from build123d import *

# Parameters (mm, degrees)
SKETCH_R  = 3
PAD_DEPTH = 5


with BuildPart() as part:
    # Sketch → Pad (new body)
    with BuildSketch(Plane.XY):
        with BuildLine():
            Line((3, 43), (3, 13))
            Line((3, 13), (-3, 13))
            Line((-3, 13), (-3, 43))
            Line((-3, 43), (-8, 43))
            ThreePointArc((-43, 8), (-18.530637, 18.530637), (-8, 43))
            Line((-43, 3), (-43, 8))
            Line((-13, 3), (-43, 3))
            Line((-13, -3), (-13, 3))
            Line((-43, -3), (-13, -3))
            Line((-43, -3), (-43, -8))
            ThreePointArc((-8, -43), (-18.530637, -18.530637), (-43, -8))
            Line((-3, -43), (-8, -43))
            Line((-3, -43), (-3, -13))
            Line((-3, -13), (3, -13))
            Line((3, -13), (3, -43))
            Line((3, -43), (8, -43))
            ThreePointArc((43, -8), (18.530637, -18.530637), (8, -43))
            Line((43, -3), (43, -8))
            Line((13, -3), (43, -3))
            Line((13, 3), (13, -3))
            Line((13, 3), (43, 3))
            Line((43, 3), (43, 8))
            ThreePointArc((8, 43), (18.530637, 18.530637), (43, 8))
            Line((3, 43), (8, 43))
        make_face()
        Circle(SKETCH_R, mode=Mode.SUBTRACT)
    extrude(amount=PAD_DEPTH)


solid = part.part
Design review of the part built by this model. Coordinates are the model's own, in mm. A direction names the side the tool comes from. Coordinates: 2 decimals unless noted, no trailing zeros. Write each loop counter-clockwise with the first axis right and the second up, starting at its lowest first coordinate (ties: lowest second). Pieces come first, ordered by that corner, then holes. Notation, with made-up numbers: (-12, -6.75) -> (29, -6.75) arc R18 cw to (29, 1.25) -> close; hole circle Ø11 at (-40, 68). An arc over 180 degrees is marked (long way). Write each question's results on one line, items separated by ' | '. Start each with the question number.
(1) Take a section at B-B on x = 0. Write out the cut boundary in (y, z).
(2) Tool access review of faces 4 (the face through (3, 28, 2)), 5 (the face through (0, -13, 2)), 6 (the face through (-28, -3, 2)), 7 (the face through (28, -3, 2)): name each direction out of +Z, -Z, +X, -X, +Y, -Y from which nothing blocks a thin tool from reaching the whole face with its end or side.
(3) The part is to be moulded in two halves that separate along Y. For faces 1 (the face through (13, 0, 2)), 2 (the face through (-18.802, 18.262, 2.465)), 3 (the face through (-18.262, -18.802, 2.465)), say which applies: pulls with the +Y half, pulls with the -Y half, needs draft (parallel to the pull), parting line crosses it, or undercut.
(4) For line 1 along Y through (x, z) = (0, 1.9); line 2 along X through (y, z) = (38, 2.8); line 3 along Y through (x, z) = (-21, 3.1), list the stretches that pass through material, from the lowest coordinate up. Write a range as from..to.
(5) Clearance check with flat-ended pins moving along their axes: P1, Ø5.5, axis at x = 0, y = 0, coming from the -Z side; P2, Ø2.5, axis at y = -28, z = 2, coming from the +X side; P3, Ø1.5, axis at y = -1, z = 3, coming from the +X side; P4, Ø1.5, axis at x = 0, z = 1.5, coming from the +Y side. State where each tip first meets the part, or that it passes through.
(6) Take a section at A-A on z = 2.2. Write out the cut boundary in (x, y), and give its area (3 significant figures).
Results found:
1) outline: (-13, 0) -> (-3, 0) -> (-3, 5) -> (-13, 5) -> close; (3, 0) -> (13, 0) -> (13, 5) -> (3, 5) -> close
2) face 4: +Z, -Z, +Y | face 5: +Z, -Z, -Y | face 6: +Z, -Z, -X | face 7: +Z, -Z, +X
3) face 1: undercut | face 2: pulls with the +Y half | face 3: pulls with the -Y half
4) line 1: y = -13..-3, 3..13 | line 2: x = -8.49..-3, 3..8.49 | line 3: y = -16.28..-3, 3..16.28
5) P1: passes through | P2: stops at x = 12.38 | P3: stops at x = 13 | P4: stops at y = 13
6) outline: (-43, -8) arc R36 cw to (-8, -43) -> (-3, -43) -> (-3, -13) -> (3, -13) -> (3, -43) -> (8, -43) arc R36 cw to (43, -8) -> (43, -3) -> (13, -3) -> (13, 3) -> (43, 3) -> (43, 8) arc R36 cw to (8, 43) -> (3, 43) -> (3, 13) -> (-3, 13) -> (-3, 43) -> (-8, 43) arc R36 cw to (-43, 8) -> (-43, 3) -> (-13, 3) -> (-13, -3) -> (-43, -3) -> close; hole circle Ø6 at (0, 0) | area: 2,860 mm2
